```python
from build123d import *

# Parameters (mm, degrees)
F0_W     = 475
F0_H     = 375
F0_R     = 55
F0_W_2   = 75.338244
F0_H_2   = 147.539295
F1_DEPTH = 25


with BuildPart() as f1:
    # F0 (on Front) → F1 (new body)
    with BuildSketch(Plane.XZ):
        Rectangle(F0_W, F0_H)
        with Locations((-100.5, 57.5)):
            Circle(F0_R, mode=Mode.SUBTRACT)
        with BuildLine():
            ThreePointArc((-12.038727, 95.723974), (34.104146, 152.384548), (87.5, 102.5))
            ThreePointArc((87.5, 102.5), (87.465172, 100.6341), (87.360737, 98.770799))
            ThreePointArc((87.360737, 98.770799), (85.927868, 90.060481), (82.985546, 81.737893))
            Line((82.985546, 81.737893), (54.449754, -29.353832))
            ThreePointArc((54.449754, -29.353832), (37.530195, -42.499974), (20.565372, -29.412296))
            Line((20.565372, -29.412296), (-9.046864, 84.241046))
            ThreePointArc((-9.046864, 84.241046), (-10.884653, 89.893439), (-12.038727, 95.723974))
        make_face(mode=Mode.SUBTRACT)
        with Locations((175.169122, 63.730353)):
            Rectangle(F0_W_2, F0_H_2, mode=Mode.SUBTRACT)
    extrude(amount=F1_DEPTH)


solid = f1.part
```
The model under review builds one solid part; all positions refer to its coordinate system, in mm. A direction names the side the tool comes from. Round coordinates to 2 decimals unless told otherwise and drop trailing zeros. Write each loop counter-clockwise with the first axis right and the second up, starting at its lowest first coordinate (ties: lowest second). Pieces come first, ordered by that corner, then holes. Notation, with made-up numbers: M -21,83.5 L 3,83.5 A28 ccw 3,114.5 Z; hole C -37.75,54.25 d9. An arc over 180 degrees is marked long. Use CSV: the item, a comma, the result in double quotes. Start each with the question number.
(1) We need section A-A, the plane x = 37.5. State the section outline as (y, z) points.
(2) We need section C-C, the plane z = 57.5. State the section outline as (x, y) points, then the cut area to 3 significant figures.
(3) We need section D-D, the plane z = -34.5. State the section outline as (x, y) points, then the cut area to 3 significant figures.
(4) Tool access review of faces 5 (the face through (-3, -25, 3)), 6 (the face through (137.5, -12, 63)): name each direction out of +Z, -Z, +X, -X, +Y, -Y from which nothing blocks a thin tool from reaching the whole face with its end or side.
(5) The part is to be moulded in two halves that separate along X. For faces 1 (the face through (-237.5, -12, -3)), 2 (the face through (5.967, -12.325, 26.619)), 3 (the face through (237.5, -12, -3)), 4 (the face through (-3, -12, -187.5)), say which applies: +X half, -X half, draft (parallel to the pull), parting line (faces both ways), or undercut.
(6) We need section B-B, the plane y = -17.5. State the section outline as (x, z) points, then the cut area to 3 significant figures.
(7) For line 1 along Z through (x, y) = (-100.5, -9.25); line 2 along X through (y, z) = (-14, 129.5); line 3 along Z through (x, y) = (168, -2.5), list the stretches that pass through material, from the lowest coordinate up.
Findings:
1,outline,"M -25,-187.5 L 0,-187.5 L 0,-42.5 L -25,-42.5 Z; M -25,152.5 L 0,152.5 L 0,187.5 L -25,187.5 Z"
2,outline,"M -237.5,-25 L -155.5,-25 L -155.5,0 L -237.5,0 Z; M -45.5,-25 L -2.08,-25 L -2.08,0 L -45.5,0 Z; M 76.76,-25 L 137.5,-25 L 137.5,0 L 76.76,0 Z; M 212.84,-25 L 237.5,-25 L 237.5,0 L 212.84,0 Z"
2,area,"5,270 mm^2"
3,outline,"M -237.5,-25 L 22.8,-25 L 22.8,0 L -237.5,0 Z; M 52.2,-25 L 237.5,-25 L 237.5,0 L 52.2,0 Z"
3,area,"11,100 mm^2"
4,face 5,"+Z, -Z, +X, -X, -Y"
4,face 6,"+Y, -Y"
5,face 1,"-X half"
5,face 2,"undercut"
5,face 3,"+X half"
5,face 4,"draft"
6,outline,"M -237.5,-187.5 L 237.5,-187.5 L 237.5,187.5 L -237.5,187.5 Z; hole C -100.5,57.5 d110; hole M -12.04,95.72 A50 ccw -9.05,84.24 L 20.57,-29.41 A17.5 ccw 54.45,-29.35 L 82.99,81.74 A50 ccw 87.36,98.77 A50 ccw 87.5,102.5 A50 ccw long Z; hole M 137.5,-10.04 L 212.84,-10.04 L 212.84,137.5 L 137.5,137.5 Z"
6,area,"144,000 mm^2"
7,line 1,"-187.5 to 2.5, 112.5 to 187.5"
7,line 2,"-237.5 to -4.58, 79.58 to 137.5, 212.84 to 237.5"
7,line 3,"-187.5 to -10.04, 137.5 to 187.5"
